Part model, mm, in its own coordinate system. A direction names the side the tool comes from. Give positions to 0.01 mm unless a question says otherwise; leave off trailing zeros. Loops run counter-clockwise (first coordinate to the right, second up) from the corner with the lowest first, then second, coordinate; pieces in that order, holes last. Notation, with made-up numbers: M -30.75,-34.75 L 1.25,-34.75 A21 cw 1.25,-27.75 Z; hole C -26.5,43 d4. An arc over 180 degrees is marked long. Answer in a Markdown table with one row per item.
from build123d import *

# Parameters (mm, degrees)
CYLINDER1391_R               = 1.5
CYLINDER1391_DEPTH           = 20
CYLINDER1390_R               = 1.5
CYLINDER1390_DEPTH           = 20
CYLINDER1385_R               = 1.5
CYLINDER1385_DEPTH           = 20
CYLINDER1389_R               = 1.5
CYLINDER1389_DEPTH           = 20
BOX514_W                     = 6
BOX514_H                     = 2
BOX514_DEPTH                 = 6
BOX511_W                     = 6
BOX511_H                     = 2
BOX511_DEPTH                 = 6
BOX513_W                     = 6
BOX513_H                     = 2
BOX513_DEPTH                 = 6
BOX512_W                     = 6
BOX512_H                     = 2
BOX512_DEPTH                 = 6
CYLINDER1392_R               = 4
CYLINDER1392_DEPTH           = 20
CYLINDER1392_PLACEMENT_ANGLE = 45
CYLINDER1387_R               = 4
CYLINDER1387_DEPTH           = 20
CYLINDER1387_PLACEMENT_ANGLE = 45
CYLINDER1384_R               = 10
CYLINDER1384_DEPTH           = 40
CYLINDER1388_R               = 10
CYLINDER1388_DEPTH           = 40
CYLINDER1386_R               = 52
CYLINDER1386_DEPTH           = 20
BOX510_W                     = 108
BOX510_H                     = 36
BOX510_DEPTH                 = 12
FILLET022_R                  = 12


with BuildPart() as obj1:
    # Cylinder1391 → Cylinder1391 (new body)
    with BuildSketch(Plane(origin=(20, -40, -5), x_dir=(1, 0, 0), z_dir=(0, -1, 0))):
        Circle(CYLINDER1391_R)
    extrude(amount=CYLINDER1391_DEPTH)


with BuildPart() as obj2:
    # Cylinder1390 → Cylinder1390 (new body)
    with BuildSketch(Plane(origin=(51, -40, 7), x_dir=(1, 0, 0), z_dir=(0, -1, 0))):
        Circle(CYLINDER1390_R)
    extrude(amount=CYLINDER1390_DEPTH)


with BuildPart() as obj3:
    # Cylinder1385 → Cylinder1385 (new body)
    with BuildSketch(Plane(origin=(-51, -40, 7), x_dir=(1, 0, 0), z_dir=(0, -1, 0))):
        Circle(CYLINDER1385_R)
    extrude(amount=CYLINDER1385_DEPTH)


with BuildPart() as compound879:
    # Cylinder1389 → Cylinder1389 (new body)
    with BuildSketch(Plane(origin=(-20, -40, -5), x_dir=(1, 0, 0), z_dir=(0, -1, 0))):
        Circle(CYLINDER1389_R)
    extrude(amount=CYLINDER1389_DEPTH)

    # Compound879: union obj1, obj2, obj3
    add(obj1.part)
    add(obj2.part)
    add(obj3.part)


with BuildPart() as krychle514:
    # Box514 → Box514 (new body)
    with BuildSketch(Plane(origin=(17, -47, -8), x_dir=(1, 0, 0), z_dir=(0, 0, 1))):
        with Locations((3, 1)):
            Rectangle(BOX514_W, BOX514_H)
    extrude(amount=BOX514_DEPTH)


with BuildPart() as krychle511:
    # Box511 → Box511 (new body)
    with BuildSketch(Plane(origin=(48, -45, 4), x_dir=(1, 0, 0), z_dir=(0, 0, 1))):
        with Locations((3, 1)):
            Rectangle(BOX511_W, BOX511_H)
    extrude(amount=BOX511_DEPTH)


with BuildPart() as krychle513:
    # Box513 → Box513 (new body)
    with BuildSketch(Plane(origin=(-54, -45, 4), x_dir=(1, 0, 0), z_dir=(0, 0, 1))):
        with Locations((3, 1)):
            Rectangle(BOX513_W, BOX513_H)
    extrude(amount=BOX513_DEPTH)


with BuildPart() as compound877:
    # Box512 → Box512 (new body)
    with BuildSketch(Plane(origin=(-23, -47, -8), x_dir=(1, 0, 0), z_dir=(0, 0, 1))):
        with Locations((3, 1)):
            Rectangle(BOX512_W, BOX512_H)
    extrude(amount=BOX512_DEPTH)

    # Compound877: union Krychle514, Krychle511, Krychle513
    add(krychle514.part)
    add(krychle511.part)
    add(krychle513.part)


with BuildPart() as obj4:
    # Cylinder1392 → Cylinder1392 (new body)
    with BuildSketch(Plane.XY):
        Circle(CYLINDER1392_R)
    extrude(amount=CYLINDER1392_DEPTH)


with BuildPart() as obj4_1:
    # Cylinder1392 placement: moved
    add(obj4.part.moved(Location((39.6, -39.6, -10))).rotate(Axis((39.6, -39.6, -10), (0, 0, 1)), CYLINDER1392_PLACEMENT_ANGLE))


with BuildPart() as compound876:
    # Cylinder1387 → Cylinder1387 (new body)
    with BuildSketch(Plane.XY):
        Circle(CYLINDER1387_R)
    extrude(amount=CYLINDER1387_DEPTH)


with BuildPart() as compound876_1:
    # Cylinder1387 placement: moved
    add(compound876.part.moved(Location((-39.6, -39.6, -10))).rotate(Axis((-39.6, -39.6, -10), (0, 0, -1)), CYLINDER1387_PLACEMENT_ANGLE))

    # Compound876: union obj4
    add(obj4_1.part)


with BuildPart() as obj5:
    # Cylinder1384 → Cylinder1384 (new body)
    with BuildSketch(Plane(origin=(-59, -17, 0), x_dir=(1, 0, 0), z_dir=(0, 0, 1))):
        Circle(CYLINDER1384_R)
    extrude(amount=CYLINDER1384_DEPTH)


with BuildPart() as compound878:
    # Cylinder1388 → Cylinder1388 (new body)
    with BuildSketch(Plane(origin=(59, -17, 0), x_dir=(1, 0, 0), z_dir=(0, 0, 1))):
        Circle(CYLINDER1388_R)
    extrude(amount=CYLINDER1388_DEPTH)

    # Compound878: union obj5
    add(obj5.part)


with BuildPart() as obj6:
    # Cylinder1386 → Cylinder1386 (new body)
    with BuildSketch(Plane.XY.offset(20)):
        Circle(CYLINDER1386_R)
    extrude(amount=CYLINDER1386_DEPTH)


with BuildPart() as fillet022:
    # Box510 → Box510 (new body)
    with BuildSketch(Plane(origin=(-54, -53, 20), x_dir=(1, 0, 0), z_dir=(0, 0, 1))):
        with Locations((54, 18)):
            Rectangle(BOX510_W, BOX510_H)
    extrude(amount=BOX510_DEPTH)

    # Cut498: cut obj6
    add(obj6.part, mode=Mode.SUBTRACT)


with BuildPart() as fillet022_1:
    # Cut498 placement: moved
    add(fillet022.part.moved(Location((0, 0, -20))))

    # Cut499: cut Compound878
    add(compound878.part, mode=Mode.SUBTRACT)

    # Cut496: cut Compound876
    add(compound876_1.part, mode=Mode.SUBTRACT)

    # Cut497: cut Compound877
    add(compound877.part, mode=Mode.SUBTRACT)

    # Cut495: cut Compound879
    add(compound879.part, mode=Mode.SUBTRACT)

    # Fillet022
    fillet022_edges = [fillet022_1.edges().sort_by_distance(p)[0] for p in [
        (-54, -25.660254, 6),
        (54, -25.660254, 6),
    ]]
    fillet(fillet022_edges, radius=FILLET022_R)


with BuildPart() as fillet022_2:
    # Fillet022 placement: moved
    add(fillet022_1.part.moved(Location((0, 0, -6))))


solid = fillet022_2.part
(1) Saw through at B-B (z = -4.5). Write the cut outline in (x, y), plus the area to 3 significant figures.
Recorded:
| item | result |
|---|---|
| outline | M -54,-53 L 54,-53 L 54,-30.96 A12 ccw 51.27,-23.35 A10 cw 49.01,-17.39 A52 cw -49.01,-17.39 A10 cw -51.27,-23.35 A12 ccw -54,-30.96 Z; hole C -39.6,-39.6 d8; hole C 39.6,-39.6 d8 |
| area | 1,210 mm^2 |
(2) Pin check, flat tips, straight feed: pin 1 Ø6.5 at (x, y) = (-39, -38) entering from -Z; pin 2 Ø1 at (x, z) = (20.5, -1.5) entering from +Y; pin 3 Ø1.8 at (x, z) = (51, 1) entering from -Y; pin 4 Ø1.6 at (y, z) = (-44, 2) entering from +X. Stop position of each tip, or through.
Recorded:
| item | result |
|---|---|
| pin 1 | stops at z = -6 |
| pin 2 | stops at y = -47.57 |
| pin 3 | stops at y = -40 |
| pin 4 | stops at x = 48 |
(3) Saw through at C-C (x = 39.6). Write the cut outline in (y, z), plus the area to 3 significant figures.
Recorded:
| item | result |
|---|---|
| outline | M -53,-6 L -43.6,-6 L -43.6,4 L -35.6,4 L -35.6,-6 L -33.7,-6 L -33.7,6 L -53,6 Z |
| area | 152 mm^2 |
(4) Drill centre lines: line 1 along Z through (x, y) = (51, -41); line 2 along X through (y, z) = (-40.75, 1); line 3 along X through (y, z) = (-42.2, 1). Where is each one in solid material? Low to high.
Recorded:
| item | result |
|---|---|
| line 1 | z = -6 to -0.5, 2.5 to 6 |
| line 2 | x = -54 to -52.5, -49.5 to -43.43, -35.77 to -32.3, 32.3 to 35.77, 43.43 to 49.5, 52.5 to 54 |
| line 3 | x = -54 to -52.5, -49.5 to -42.64, -36.56 to -30.38, 30.38 to 36.56, 42.64 to 49.5, 52.5 to 54 |
(5) Which spindle directions (+Z, -Z, +X, -X, +Y, -Y) get a long thin tool onto all of the face, cutting with end or side? Do faces 5 (the face through (-13, -51, 6)), 6 (the face through (51, -44, 4)), 7 (the face through (54, -42, 0)), 8 (the face through (49.5, -41.48, 1.07)), 9 (the face through (-52.4, -43, -0.4)). Say none if no direction does.
Recorded:
| item | result |
|---|---|
| face 5 | +Z, +X, -X, +Y, -Y |
| face 6 | +X |
| face 7 | +Z, -Z, +X, +Y, -Y |
| face 8 | -Y |
| face 9 | -X |
(6) Saw through at A-A (z = 1). Give the number of separate pieces and of enclosed holes in the cut face, plus the area to 3 significant figures.
Recorded:
| item | result |
|---|---|
| separate pieces | 3 |
| enclosed holes | 2 |
| area | 1,120 mm^2 |
(7) Pull direction X, two halves, no side cores. Call faces 1 (the face through (-51, -44, 4)), 2 (the face through (51, -40, 1)), 3 (the face through (-49.668, -20.595, -0.084)), 4 (the face through (49.5, -48.94, 1.07)): +X half, -X half, draft (parallel to the pull), parting line (faces both ways), or undercut.
Recorded:
| item | result |
|---|---|
| face 1 | draft |
| face 2 | undercut |
| face 3 | -X half |
| face 4 | undercut |
(8) Saw through at D-D (x = -18.5). Write the cut outline in (y, z).
Recorded:
| item | result |
|---|---|
| outline | M -53,-6 L -48.6,-6 L -48.6,6 L -53,6 Z |
